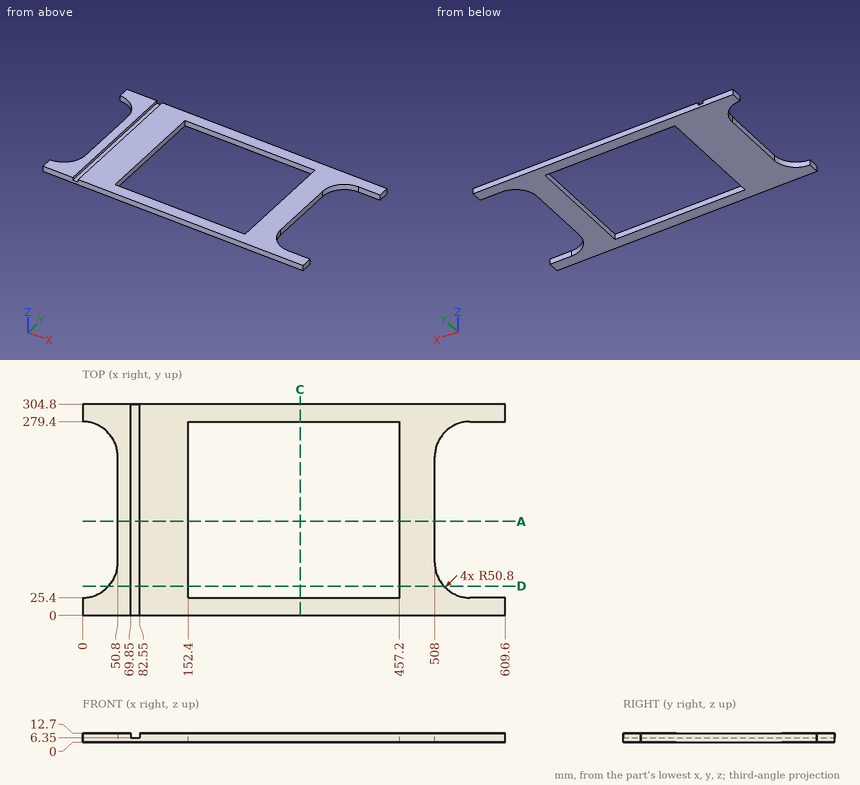
Part print with two shaded views. Sizes in mm from the minimum x, y, z corner. Round coordinates to 2 decimals unless told otherwise and drop trailing zeros. Order: outer loops, then holes, each group sorted by start corner. A loop starts at its lowest first (then second) coordinate and runs counter-clockwise, first axis right, second up. Notation, with made-up numbers: M 29,38.5 L 79,38.5 A23 ccw 79,69.5 Z; hole C -19,-17 d11. An arc over 180 degrees is marked long. Use CSV: the item, a comma, the result in double quotes.
Item 1: Saw through at A-A (y = 135.5). List the corners of the cut face in (x, z).
Worked answers:
outline,"M 50.8,0 L 152.4,0 L 152.4,12.7 L 82.55,12.7 L 82.55,6.35 L 69.85,6.35 L 69.85,12.7 L 50.8,12.7 Z; M 457.2,0 L 508,0 L 508,12.7 L 457.2,12.7 Z"
Item 2: Pin check, flat tips, straight feed: pin 1 (2 mm diameter, centred on y = 229.5, z = 2.5, fed in from +X); pin 2 (3 mm diameter, centred on x = 238, z = 6, fed in from -Y); pin 3 (3 mm diameter, centred on y = 43.5, z = 7.5, fed in from +X); pin 4 (5 mm diameter, centred on y = 222, z = 8.5, fed in from -X). Stop position of each tip, or through.
Worked answers:
pin 1,"x = 508.04"
pin 2,"y = 0"
pin 3,"x = 521.24"
pin 4,"x = 50.8"
Item 3: Probe probe 1 along X at (y, z) = (167, 6.75); probe 2 along X at (y, z) = (13, 7.5); probe 3 along Y at (x, z) = (294, 8). List the from-to ranges inside material, lowest first.
Worked answers:
probe 1,"50.8 to 69.85, 82.55 to 152.4, 457.2 to 508"
probe 2,"0 to 69.85, 82.55 to 609.6"
probe 3,"0 to 25.4, 279.4 to 304.8"
Item 4: Saw through at D-D (y = 42). List the corners of the cut face in (x, z), plus the area to 3 significant figures.
Worked answers:
outline,"M 37.56,0 L 152.4,0 L 152.4,12.7 L 82.55,12.7 L 82.55,6.35 L 69.85,6.35 L 69.85,12.7 L 37.56,12.7 Z; M 457.2,0 L 521.24,0 L 521.24,12.7 L 457.2,12.7 Z"
area,"2,190 mm²"
Item 5: Saw through at C-C (x = 314). List the corners of the cut face in (y, z), plus the area to 3 significant figures.
Worked answers:
outline,"M 0,0 L 25.4,0 L 25.4,12.7 L 0,12.7 Z; M 279.4,0 L 304.8,0 L 304.8,12.7 L 279.4,12.7 Z"
area,"645 mm²"
